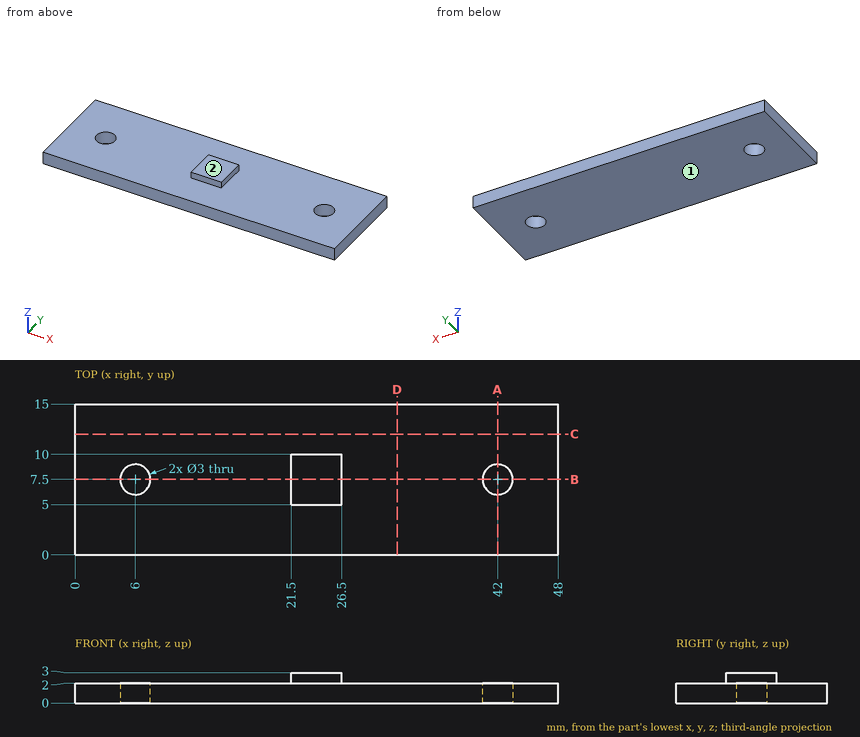
The drawing under review shows one solid part. Ordinate dimensions are in mm from its lowest x, y, z. Round coordinates to 2 decimals unless told otherwise and drop trailing zeros. Write each loop counter-clockwise with the first axis right and the second up, starting at its lowest first coordinate (ties: lowest second). Pieces come first, ordered by that corner, then holes.
(1) Insertion check: pin 1 (4.5 mm diameter, centred on x = 32, y = 8, fed in from +Z); pin 2 (0.8 mm diameter, centred on y = 7.5, z = 2.5, fed in from -X); pin 3 (0.5 mm diameter, centred on x = 24.5, z = 2.5, fed in from -Y). Each pin has a flat end and moves straight along its axis. Give the tip position at first contact, or say it passes through.
(2) We need section D-D on x = 32. Give the boundary of the cut face in (y, z).
(3) We need section B-B on y = 7.5. Give the boundary of the cut face in (x, z), and give its area (3 significant figures).
(4) We need section A-A on x = 42. Give the boundary of the cut face in (y, z), and give its area (3 significant figures).
(5) We need section C-C on y = 12. Give the boundary of the cut face in (x, z), and give its area (3 significant figures).
(6) Mouldability with a two-part tool opening along Z and no side actions: class the marked faces 1 and 2 as +Z half, -Z half, draft (parallel to the pull), parting line (faces both ways), or undercut.
(7) Wall thickness on L1, parallel to Y at x = 6, z = 1.5; L2, parallel to Z at x = 4, y = 9.25; L3, parallel to Y at x = 23.5, z = 2.9: over which ranges is each line inside the solid? List them lowest first.
Findings below:
1. pin 1: stops at z = 2
1. pin 2: stops at x = 21.5
1. pin 3: stops at y = 5
2. outline: (0, 0) - (15, 0) - (15, 2) - (0, 2) - close
3. outline: (0, 0) - (4.5, 0) - (4.5, 2) - (0, 2) - close; (7.5, 0) - (40.5, 0) - (40.5, 2) - (26.5, 2) - (26.5, 3) - (21.5, 3) - (21.5, 2) - (7.5, 2) - close; (43.5, 0) - (48, 0) - (48, 2) - (43.5, 2) - close
3. area: 89.0 mm2
4. outline: (0, 0) - (6, 0) - (6, 2) - (0, 2) - close; (9, 0) - (15, 0) - (15, 2) - (9, 2) - close
4. area: 24.0 mm2
5. outline: (0, 0) - (48, 0) - (48, 2) - (0, 2) - close
5. area: 96.0 mm2
6. face 1: -Z half
6. face 2: +Z half
7. L1: y = 0 to 6, 9 to 15
7. L2: z = 0 to 2
7. L3: y = 5 to 10
